from build123d import *

# Parameters (mm, degrees)
F0_W       = 127
F0_H       = 76.2
F1_DEPTH   = 9.525
F3_DEPTH   = 3.175
F4_W       = 127
F4_H       = 38.1
F5_DEPTH   = 19.05
F6_W       = 50.8
F6_H       = 38.1
F7_DEPTH   = 38.1
F9_D       = 9.525
F10_R      = 9.525
F10_R_2    = 4.7625
F11_DEPTH  = 12.7
F12_R      = 9.525
F12_R_2    = 4.7625
F13_DEPTH  = 12.7
F17_R      = 12.7
F7_FACE_R  = 9.525
F18_DEPTH  = 2.54
F15_R      = 12.7
F7_FACE1_R = 9.525
F19_DEPTH  = 2.54
F20_R      = 12.7
F21_R      = 12.7


with BuildPart() as f1:
    # F0 (on Front) → F1 (new body)
    with BuildSketch(Plane.XZ):
        with Locations((0.997369945, 3.3350293577)):
            Rectangle(F0_W, F0_H)
        with BuildLine():
            ThreePointArc((-33.927630055, -28.4149706423), (-37.102630055, -25.2399706423), (-33.927630055, -22.0649706423))
            Line((-33.927630055, -22.0649706423), (39.097369945, -22.0649706423))
            ThreePointArc((39.097369945, -22.0649706423), (42.272369945, -25.2399706423), (39.097369945, -28.4149706423))
            Line((39.097369945, -28.4149706423), (-33.927630055, -28.4149706423))
        make_face(mode=Mode.SUBTRACT)
        with BuildLine():
            Line((39.097369945, 28.2236666642), (-33.927630055, 28.2236666642))
            ThreePointArc((-33.927630055, 28.2236666642), (-37.102630055, 31.3986666642), (-33.927630055, 34.5736666642))
            Line((-33.927630055, 34.5736666642), (39.097369945, 34.5736666642))
            ThreePointArc((39.097369945, 34.5736666642), (42.272369945, 31.3986666642), (39.097369945, 28.2236666642))
        make_face(mode=Mode.SUBTRACT)
    extrude(amount=F1_DEPTH)

    # F2 (on face) → F3 (cut)
    with BuildSketch(Plane.XZ.offset(9.525)):
        with BuildLine():
            Line((39.097369945, -18.8899706423), (-33.927630055, -18.8899706423))
            ThreePointArc((-33.927630055, -18.8899706423), (-40.277630055, -25.2399706423), (-33.927630055, -31.5899706423))
            Line((-33.927630055, -31.5899706423), (39.097369945, -31.5899706423))
            ThreePointArc((39.097369945, -31.5899706423), (45.447369945, -25.2399706423), (39.097369945, -18.8899706423))
        make_face()
        with BuildLine():
            Line((39.097369945, -28.4149706423), (-33.927630055, -28.4149706423))
            ThreePointArc((-33.927630055, -28.4149706423), (-37.102630055, -25.2399706423), (-33.927630055, -22.0649706423))
            Line((-33.927630055, -22.0649706423), (39.097369945, -22.0649706423))
            ThreePointArc((39.097369945, -22.0649706423), (42.272369945, -25.2399706423), (39.097369945, -28.4149706423))
        make_face(mode=Mode.SUBTRACT)
        with BuildLine():
            ThreePointArc((-33.927630055, 38.2600293577), (-40.277630055, 31.9100293577), (-33.927630055, 25.5600293577))
            Line((-33.927630055, 25.5600293577), (39.097369945, 25.5600293577))
            ThreePointArc((39.097369945, 25.5600293577), (45.447369945, 31.9100293577), (39.097369945, 38.2600293577))
            Line((39.097369945, 38.2600293577), (-33.927630055, 38.2600293577))
        make_face()
        with BuildLine():
            Line((-33.927630055, 34.5736666642), (39.097369945, 34.5736666642))
            ThreePointArc((39.097369945, 34.5736666642), (42.272369945, 31.3986666642), (39.097369945, 28.2236666642))
            Line((39.097369945, 28.2236666642), (-33.927630055, 28.2236666642))
            ThreePointArc((-33.927630055, 28.2236666642), (-37.102630055, 31.3986666642), (-33.927630055, 34.5736666642))
        make_face(mode=Mode.SUBTRACT)
    extrude(amount=-F3_DEPTH, mode=Mode.SUBTRACT)

    # F4 (on face) → F5 (join)
    with BuildSketch(Plane.XZ.offset(9.525)):
        with Locations((0.997369945, 3.3350293577)):
            Rectangle(F4_W, F4_H)
    extrude(amount=F5_DEPTH)

    # F6 (on face) → F7 (join)
    with BuildSketch(Plane.XZ.offset(28.575)):
        with Locations((0.997369945, 3.3350293577)):
            Rectangle(F6_W, F6_H)
    extrude(amount=F7_DEPTH)

    # F9 (through all)
    with Locations(Plane(origin=(0, 0, -15.7149706423), x_dir=(1, 0, 0), z_dir=(0, 0, -1))):
        with Locations((0.997369945, 47.625)):
            Hole(F9_D / 2)

    # F10 (on face) → F11 (cut)
    with BuildSketch(Plane(origin=(0, 0, -15.7149706423), x_dir=(1, 0, 0), z_dir=(0, 0, -1))):
        with Locations((0.997369945, 47.625)):
            Circle(F10_R)
        with Locations((0.997369945, 47.625)):
            Circle(F10_R_2, mode=Mode.SUBTRACT)
    extrude(amount=-F11_DEPTH, mode=Mode.SUBTRACT)

    # F12 (on face) → F13 (cut)
    with BuildSketch(Plane.XY.offset(22.3850293577)):
        with Locations((0.997369945, -47.625)):
            Circle(F12_R)
        with Locations((0.997369945, -47.625)):
            Circle(F12_R_2, mode=Mode.SUBTRACT)
        with Locations((0.997369945, -47.625)):
            Circle(F12_R)
    extrude(amount=-F13_DEPTH, mode=Mode.SUBTRACT)

    # F17 (on offset) + F7_face (on face) → F18 (cut)
    with BuildSketch(Plane(origin=(0, 0, -10.6349706423), x_dir=(1, 0, 0), z_dir=(0, 0, -1))):
        with Locations((0.997369945, 47.625)):
            Circle(F17_R)
    with BuildSketch(Plane(origin=(0.997369945, -31.75, -15.7149706423), x_dir=(1, 0, 0), z_dir=(0, 0, -1))):
        Polygon((-63.5, -3.175), (-63.5, -22.225), (63.5, -22.225), (63.5, -3.175), (25.4, -3.175), (25.4, 34.925), (-25.4, 34.925), (-25.4, -3.175), align=None)
        with Locations((0, 15.875)):
            Circle(F7_FACE_R, mode=Mode.SUBTRACT)
    extrude(amount=F18_DEPTH, mode=Mode.SUBTRACT)

    # F15 (on offset) + F7_face1 (on face) → F19 (cut)
    with BuildSketch(Plane.XY.offset(17.3050293577)):
        with Locations((0.997369945, -47.625)):
            Circle(F15_R)
    with BuildSketch(Plane(origin=(0.997369945, -31.4859250029, 22.3850293577), x_dir=(1, 0, 0), z_dir=(0, 0, 1))):
        Polygon((63.5, 2.9109250029), (63.5, 21.9609250029), (-63.5, 21.9609250029), (-63.5, 2.9109250029), (-25.4, 2.9109250029), (-25.4, -35.1890749971), (25.4, -35.1890749971), (25.4, 2.9109250029), align=None)
        with Locations((0, -16.1390749971)):
            Circle(F7_FACE1_R, mode=Mode.SUBTRACT)
    extrude(amount=F19_DEPTH, mode=Mode.SUBTRACT)

    # F20
    f20_edges = [f1.edges().sort_by_distance(p)[0] for p in [
        (-62.50263, -28.575, 3.335029),
        (-24.40263, -28.575, 3.335029),
        (-24.40263, -66.675, 3.335029),
        (26.39737, -66.675, 3.335029),
        (26.39737, -28.575, 3.335029),
    ]]
    fillet(f20_edges, radius=F20_R)

    # F21
    f21_edges = [f1.edges().sort_by_distance(p)[0] for p in [
        (64.49737, -28.575, 3.335029),
    ]]
    fillet(f21_edges, radius=F21_R)


solid = f1.part
Input: part model. Units: mm. Frame: model coordinates. A direction names the side the tool comes from. Round coordinates to 2 decimals unless told otherwise and drop trailing zeros. Write each loop counter-clockwise with the first axis right and the second up, starting at its lowest first coordinate (ties: lowest second). Pieces come first, ordered by that corner, then holes.
1) Draft query along Y for faces 6 (the cylindrical face through (6.86, -58.89, 18.56)), 7 (the cylindrical face through (-28.024, -32.394, 3.602)), 8 (the flat face through (2, -3, -22.065)), 9 (the flat face through (6, -56, -13.175)). Return one class per face: pulls with the +Y half, pulls with the -Y half, needs draft (parallel to the pull), parting line crosses it, or undercut.
2) Ray query, L1, parallel to Z at x = -9, y = -46; L2, parallel to Z at x = 17.5, y = -4.5; L3, parallel to Z at x = 22, y = -18. Return the intervals inside material, ascending.
3) Cut plane D-D (x = 29.5). Return the cut outline in (y, z) (3 decimals), then the cut area to 3 significant figures.
4) Cut plane C-C (z = 14.5). Return the cut outline in (x, y) (3 decimals).
5) Cut plane A-A (x = -27). Return the cut outline in (y, z) (3 decimals).
6) Reachability of faces 1 (the cylindrical face through (-1.067, -38.327, -14.463)), 2 (the flat face through (3, -3, -28.415)), 3 (the cylindrical face through (-1.067, -56.923, 21.133)), 4 (the cylindrical face through (-58.881, -24.756, 3.602)), 5 (the cylindrical face through (-40.276, -7.96, 32.05)) from +Z, -Z, +X, -X, +Y, -Y: full face, straight path, thin tool, end or side. Return the list, or none.
7) Cut plane B-B (y = -3.5). Return the cut outline in (x, z) (3 decimals).
8) Contact query for flat-ended pins moving along their axis: P1, Ø22, axis at x = 1, y = -47.62, coming from the -Z side (3 decimals); P2, Ø3, axis at x = 46.5, z = 9.5, coming from the +Y side; P3, Ø15, axis at x = 1, y = -47.62, coming from the +Z side (3 decimals); P4, Ø21, axis at x = 5.5, y = -47, coming from the +Z side (3 decimals). Output: stop coordinate, or through.
Geometry says:
1. face 6: undercut
1. face 7: pulls with the -Y half
1. face 8: needs draft
1. face 9: undercut
2. L1: z = -15.71 to -13.17, -10.63 to 17.31, 19.85 to 22.39
2. L2: z = -34.76 to -28.41, -22.06 to 28.22, 34.57 to 41.44
2. L3: z = -15.71 to 22.39
3. outline: (-32.958, -15.715) - (-9.525, -15.715) - (-9.525, -18.89) - (-6.35, -18.89) - (-6.35, -22.065) - (0, -22.065) - (0, 28.224) - (-6.35, 28.224) - (-6.35, 25.56) - (-9.525, 25.56) - (-9.525, 22.385) - (-32.958, 22.385) - close; (-9.525, -34.765) - (0, -34.765) - (0, -28.415) - (-6.35, -28.415) - (-6.35, -31.59) - (-9.525, -31.59) - close; (-9.525, 38.26) - (-6.35, 38.26) - (-6.35, 34.574) - (0, 34.574) - (0, 41.435) - (-9.525, 41.435) - close
3. area: 1,460 mm2
4. outline: (-62.503, -15.875) arc R12.7 ccw to (-49.803, -28.575) - (-37.103, -28.575) arc R12.7 cw to (-24.403, -41.275) - (-24.403, -53.975) arc R12.7 ccw to (-11.703, -66.675) - (13.697, -66.675) arc R12.7 ccw to (26.397, -53.975) - (26.397, -41.275) arc R12.7 cw to (39.097, -28.575) - (51.797, -28.575) arc R12.7 ccw to (64.497, -15.875) - (64.497, 0) - (-62.503, 0) - close; hole circle Ø19.05 at (0.997, -47.625)
5. outline: (-33.579, -15.715) - (-9.525, -15.715) - (-9.525, -18.89) - (-6.35, -18.89) - (-6.35, -22.065) - (0, -22.065) - (0, 28.224) - (-6.35, 28.224) - (-6.35, 25.56) - (-9.525, 25.56) - (-9.525, 22.385) - (-33.579, 22.385) - close; (-9.525, -34.765) - (0, -34.765) - (0, -28.415) - (-6.35, -28.415) - (-6.35, -31.59) - (-9.525, -31.59) - close; (-9.525, 38.26) - (-6.35, 38.26) - (-6.35, 34.574) - (0, 34.574) - (0, 41.435) - (-9.525, 41.435) - close
6. face 1: -Z
6. face 2: +Y, -Y
6. face 3: +Z
6. face 4: +Z, -Z, -X, -Y
6. face 5: -Y
7. outline: (-62.503, -34.765) - (64.497, -34.765) - (64.497, 41.435) - (-62.503, 41.435) - close; hole (-33.928, -28.415) - (39.097, -28.415) arc R3.175 ccw to (39.097, -22.065) - (-33.928, -22.065) arc R3.175 ccw to start; hole (-33.928, 28.224) - (39.097, 28.224) arc R3.175 ccw to (39.097, 34.574) - (-33.928, 34.574) arc R3.175 ccw to start
8. P1: stops at z = -15.715
8. P2: stops at y = 0
8. P3: stops at z = 9.685
8. P4: stops at z = 22.385
